from build123d import *

# Parameters (mm, degrees)
ESQUISSE1_W             = 34
ESQUISSE1_H             = 40
BOSS_EXTRU_1_DEPTH      = 3
ESQUISSE2_R             = 6.5
ENL_V_MAT_EXTRU_1_DEPTH = 4
ESQUISSE5_R             = 1.5
ENL_V_MAT_EXTRU_3_DEPTH = 5
ESQUISSE9_W             = 34
ESQUISSE9_H             = 5
BOSS_EXTRU_5_DEPTH      = 5
ESQUISSE10_R            = 1.5
ENL_V_MAT_EXTRU_6_DEPTH = 54.103672189
ESQUISSE11_W            = 3
ESQUISSE11_H            = 30
BOSS_EXTRU_6_DEPTH      = 5
ESQUISSE12_R            = 1.5
ENL_V_MAT_EXTRU_7_DEPTH = 5
CHANFREIN1_SIZE         = 0.5


with BuildPart() as part:
    # Esquisse1 → Boss.-Extru.1 (new body)
    with BuildSketch(Plane.XY):
        with Locations((17, 20)):
            Rectangle(ESQUISSE1_W, ESQUISSE1_H)
    extrude(amount=BOSS_EXTRU_1_DEPTH)

    # Esquisse2 → Enlèv. mat.-Extru.1 (cut)
    with BuildSketch(Plane.XY.offset(3)):
        with Locations((15.5, 20)):
            Circle(ESQUISSE2_R)
    extrude(amount=-ENL_V_MAT_EXTRU_1_DEPTH, mode=Mode.SUBTRACT)

    # Esquisse5 → Enlèv. mat.-Extru.3 (cut)
    with BuildSketch(Plane.XY.offset(3)):
        with Locations((15.5, 30)):
            Circle(ESQUISSE5_R)
        with Locations((5.5, 20)):
            Circle(ESQUISSE5_R)
        with Locations((15.5, 10)):
            Circle(ESQUISSE5_R)
        with Locations((25.5, 20)):
            Circle(ESQUISSE5_R)
    extrude(amount=-ENL_V_MAT_EXTRU_3_DEPTH, mode=Mode.SUBTRACT)

    # Esquisse9 → Boss.-Extru.5 (add)
    with BuildSketch(Plane.XY.offset(3)):
        with Locations((17, 37.5)):
            Rectangle(ESQUISSE9_W, ESQUISSE9_H)
        with Locations((17, 2.5)):
            Rectangle(ESQUISSE9_W, ESQUISSE9_H)
    extrude(amount=BOSS_EXTRU_5_DEPTH)

    # Esquisse10 → Enlèv. mat.-Extru.6 (cut, through all)
    with BuildSketch(Plane(origin=(34, 0, 0), x_dir=(0, 0, -1), z_dir=(1, 0, 0))):
        with Locations((-5.5, 37.5)):
            Circle(ESQUISSE10_R)
        with Locations(Location((-5.5, 2.5, 0), (0, 0, 180))):
            Circle(ESQUISSE10_R)
    extrude(amount=-ENL_V_MAT_EXTRU_6_DEPTH, mode=Mode.SUBTRACT)

    # Esquisse11 → Boss.-Extru.6 (add)
    with BuildSketch(Plane.XY.offset(3)):
        with Locations((32.5, 20)):
            Rectangle(ESQUISSE11_W, ESQUISSE11_H)
    extrude(amount=BOSS_EXTRU_6_DEPTH)

    # Esquisse12 → Enlèv. mat.-Extru.7 (cut)
    with BuildSketch(Plane(origin=(34, 0, 0), x_dir=(0, 0, -1), z_dir=(1, 0, 0))):
        with Locations((-5.5, 20)):
            Circle(ESQUISSE12_R)
    extrude(amount=-ENL_V_MAT_EXTRU_7_DEPTH, mode=Mode.SUBTRACT)

    # Chanfrein1
    chanfrein1_edges = [part.edges().sort_by_distance(p)[0] for p in [
        (9, 20, 0),
        (9, 20, 3),
        (14, 30, 0),
        (14, 30, 3),
        (4, 20, 0),
        (4, 20, 3),
        (14, 10, 0),
        (14, 10, 3),
        (24, 20, 0),
        (24, 20, 3),
        (0, 20, 3),
        (15.5, 35, 3),
        (0, 35, 5.5),
        (0, 37.5, 8),
        (15.5, 35, 8),
        (34, 20, 8),
        (17, 40, 8),
        (17, 40, 0),
        (34, 20, 0),
        (0, 5, 5.5),
        (17, 0, 0),
        (0, 2.5, 8),
        (17, 0, 8),
        (0, 20, 0),
        (0, 37.5, 7),
        (34, 37.5, 7),
        (0, 2.5, 4),
        (34, 2.5, 4),
        (0, 40, 4),
        (15.5, 5, 8),
        (15.5, 5, 3),
        (34, 40, 4),
        (34, 0, 4),
        (0, 0, 4),
        (31, 20, 3),
        (31, 35, 5.5),
        (31, 5, 5.5),
        (31, 20, 8),
        (31, 20, 7),
        (34, 20, 7),
    ]]
    chamfer(chanfrein1_edges, length=CHANFREIN1_SIZE - 0.0001)  # a hair under: the kernel refuses the full size


solid = part.part
Work out the finished part from the listing and answer in its coordinate system (mm). A direction names the side the tool comes from. Round coordinates to 2 decimals unless told otherwise and drop trailing zeros. Write each loop counter-clockwise with the first axis right and the second up, starting at its lowest first coordinate (ties: lowest second). Pieces come first, ordered by that corner, then holes. Notation, with made-up numbers: (53.25, 5.5) - (95.25, 5.5) arc R16 cw to (95.25, 13.5) - close; hole circle Ø7 at (2, 70.25). An arc over 180 degrees is marked (long way). Answer in a Markdown table with one row per item. Add a question column.
1. The mould has two halves that part along X. Classify faces 3 (the cylindrical face through (32.51, 21.01, 6.61)), 4 (the cylindrical face through (10.709, 24.393, 1.514)), 5 (the cylindrical face through (24.39, 21.01, 1.51)): +X half, -X half, draft (parallel to the pull), parting line (faces both ways), or undercut.
2. A cutting plane is placed at D-D, the plane x = 15.5. Count the separate pieces of the cut face and the enclosed holes in it, and give its area (3 significant figures).
3. Find the intervals of material crossed by line 1 along Y through (x, z) = (15.5, 2.15); line 2 along Y through (x, z) = (25.5, 1.45); line 3 along Z through (x, y) = (11.5, 2.5), in increasing order. Write a range as from..to.
4. A cutting plane is placed at C-C, the plane z = 1.75. Determine the outline of the cut face in (x, y), and give its area (3 significant figures).
5. Given pin 1 (1.5 mm diameter, centred on y = 29.5, z = 5, fed in from -X); pin 2 (3.5 mm diameter, centred on x = 15.5, y = 30, fed in from -Z); pin 3 (12 mm diameter, centred on x = 17.5, y = 22, fed in from +Z), each flat-ended and moving along its own axis, determine where each tip first touches the part or whether it passes through.
6. A cutting plane is placed at B-B, the plane x = 2.5. Determine the outline of the cut face in (y, z), and give its area (3 significant figures).
7. For faces 1 (the cylindrical face through (17.231, 36.036, 5.825)), 2 (the flat face through (12, 27, 3)), determine the directions among +Z, -Z, +X, -X, +Y, -Y from which every point of the face is accessible in a straight line to the end or side of a thin tool.
Worked out:
| question | item | result |
|---|---|---|
| 1 | face 3 | draft |
| 1 | face 4 | undercut |
| 1 | face 5 | undercut |
| 2 | separate pieces | 4 |
| 2 | enclosed holes | 2 |
| 2 | area | 96.9 mm^2 |
| 3 | line 1 | 0..8.5, 11.5..13.5, 26.5..28.5, 31.5..40 |
| 3 | line 2 | 0..18.5, 21.5..40 |
| 3 | line 3 | 0..4, 7..8 |
| 4 | outline | (0, 0.5) - (0.5, 0) - (33.5, 0) - (34, 0.5) - (34, 39.5) - (33.5, 40) - (0.5, 40) - (0, 39.5) - close; hole circle Ø3 at (5.5, 20); hole circle Ø13 at (15.5, 20); hole circle Ø3 at (15.5, 10); hole circle Ø3 at (15.5, 30); hole circle Ø3 at (25.5, 20) |
| 4 | area | 1,200 mm^2 |
| 5 | pin 1 | x = 31 |
| 5 | pin 2 | z = 0.25 |
| 5 | pin 3 | z = 3 |
| 6 | outline | (0, 0.5) - (0.5, 0) - (39.5, 0) - (40, 0.5) - (40, 7.5) - (39.5, 8) - (35.5, 8) - (35, 7.5) - (35, 3.5) - (34.5, 3) - (5.5, 3) - (5, 3.5) - (5, 7.5) - (4.5, 8) - (0.5, 8) - (0, 7.5) - close; hole circle Ø3 at (2.5, 5.5); hole circle Ø3 at (37.5, 5.5) |
| 6 | area | 155 mm^2 |
| 7 | face 1 | +X, -X |
| 7 | face 2 | +Z, -X |
